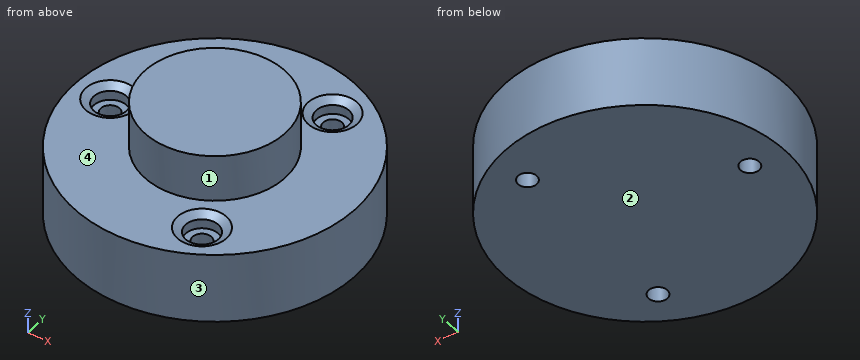
```python
from build123d import *

# Parameters (mm, degrees)
F0_R       = 30
F0_R_2     = 3.5
F0_R_3     = 15
F1_DEPTH   = 15
F2_DEPTH   = 25
F0_R_4     = 2
F3_DEPTH   = 12
F4_SIZE2   = 1.7320508076
F4_SIZE    = 1
F4_2_SIZE2 = 1.7320508076
F4_2_SIZE  = 1
F4_3_SIZE2 = 1.7320508076
F4_3_SIZE  = 1


with BuildPart() as f1:
    # F0 (on Top) → F1 (new body)
    with BuildSketch(Plane.XY):
        Circle(F0_R)
        with Locations((11.25, -19.4855715851)):
            Circle(F0_R_2, mode=Mode.SUBTRACT)
        with Locations((-22.5, 0)):
            Circle(F0_R_2, mode=Mode.SUBTRACT)
        Circle(F0_R_3, mode=Mode.SUBTRACT)
        with Locations((11.25, 19.4855715851)):
            Circle(F0_R_2, mode=Mode.SUBTRACT)
    extrude(amount=F1_DEPTH)

    # F0 (on Top) → F2 (join)
    with BuildSketch(Plane.XY):
        Circle(F0_R_3)
    extrude(amount=F2_DEPTH)

    # F0 (on Top) → F3 (join)
    with BuildSketch(Plane.XY):
        with Locations((11.25, 19.4855715851)):
            Circle(F0_R_2)
        with Locations((11.25, 19.4855715851)):
            Circle(F0_R_4, mode=Mode.SUBTRACT)
        with Locations((11.25, -19.4855715851)):
            Circle(F0_R_2)
        with Locations((11.25, -19.4855715851)):
            Circle(F0_R_4, mode=Mode.SUBTRACT)
        with Locations((-22.5, 0)):
            Circle(F0_R_2)
        with Locations((-22.5, 0)):
            Circle(F0_R_4, mode=Mode.SUBTRACT)
    extrude(amount=F3_DEPTH)

    # F4
    f4_edges = [f1.edges().sort_by_distance(p)[0] for p in [
        (-26, 0, 15),
    ]]
    f4_side = f1.faces().sort_by_distance((-26, 0, 13.5))[0]
    chamfer(f4_edges, length=F4_SIZE, length2=F4_SIZE2, reference=f4_side)

    # F4#2
    f4_2_edges = [f1.edges().sort_by_distance(p)[0] for p in [
        (7.75, -19.485572, 15),
    ]]
    f4_2_side = f1.faces().sort_by_distance((7.75, -19.485572, 13.5))[0]
    chamfer(f4_2_edges, length=F4_2_SIZE, length2=F4_2_SIZE2, reference=f4_2_side)

    # F4#3
    f4_3_edges = [f1.edges().sort_by_distance(p)[0] for p in [
        (7.75, 19.485572, 15),
    ]]
    f4_3_side = f1.faces().sort_by_distance((7.75, 19.485572, 13.5))[0]
    chamfer(f4_3_edges, length=F4_3_SIZE, length2=F4_3_SIZE2, reference=f4_3_side)


solid = f1.part
```
Source: CAD feature listing. Evaluate the final solid. Frame: model axes, mm. Face numbers are marked on the shaded views. A direction names the side the tool comes from. Coordinates: 2 decimals unless noted, no trailing zeros. Loops run counter-clockwise (first coordinate to the right, second up) from the corner with the lowest first, then second, coordinate; pieces in that order, holes last. Notation, with made-up numbers: M -10,25.5 L 15,25.5 A31 ccw 15,51.5 Z; hole C -4,64.25 d10. An arc over 180 degrees is marked long. Put each result on its own line as item: value. Start each with the question number.
1) Pull-direction query (Y, two-part tool) for the marked faces 3 and 4; classes: pulls with the +Y half, pulls with the -Y half, needs draft (parallel to the pull), parting line crosses it, or undercut.
2) Cut plane C-C on x = -22.5. Return the cut outline in (y, z), then the cut area to 3 significant figures.
3) Cut plane A-A on y = 0. Return the cut outline in (x, z).
4) Cut plane B-B on x = 0. Return the cut outline in (y, z).
5) Cut plane D-D on z = 17.75. Return the cut outline in (x, y), then the cut area to 3 significant figures.
6) Reachability of the marked faces 1 and 2 from +Z, -Z, +X, -X, +Y, -Y: full face, straight path, thin tool, end or side. Return the list, or none.
7) Ray query, L1, parallel to Y at x = 10, z = 13.25; L2, parallel to Y at x = 11.25, z = 6.5; L3, parallel to Z at x = 10, y = 13.5. Return the intervals inside material, ascending. Write a range as from..to.
8) Contact query for flat-ended pins moving along their axis: pin 1 Ø7.5 at (x, y) = (12.5, -21) entering from +Z; pin 2 Ø10 at (x, z) = (-1, 13) entering from +Y; pin 3 Ø4.5 at (x, y) = (11.25, 19.49) entering from +Z; pin 4 Ø3.5 at (x, y) = (11.25, -19.49) entering from +Z. Output: stop coordinate, or through.
The answers:
1. face 3: parting line crosses it
1. face 4: needs draft
2. outline: M -19.84,0 L -2,0 L -2,12 L -3.5,12 L -3.5,14 L -5.23,15 L -19.84,15 Z; M 2,0 L 19.84,0 L 19.84,15 L 5.23,15 L 3.5,14 L 3.5,12 L 2,12 Z
2. area: 525 mm²
3. outline: M -30,0 L -24.5,0 L -24.5,12 L -26,12 L -26,14 L -27.73,15 L -30,15 Z; M -20.5,0 L 30,0 L 30,15 L 15,15 L 15,25 L -15,25 L -15,15 L -17.27,15 L -19,14 L -19,12 L -20.5,12 Z
4. outline: M -30,0 L 30,0 L 30,15 L 15,15 L 15,25 L -15,25 L -15,15 L -30,15 Z
5. outline: C 0,0 d30
5. area: 707 mm²
6. face 1: +Z
6. face 2: -Z, +X, -X, +Y, -Y
7. L1: y = -28.28..-22.75, -16.22..16.22, 22.75..28.28
7. L2: y = -27.81..-21.49, -17.49..17.49, 21.49..27.81
7. L3: z = 0..15
8. pin 1: stops at z = 15
8. pin 2: stops at y = 30
8. pin 3: stops at z = 12
8. pin 4: passes through
